Could you check a few things on this model? Use its own coordinates, in mm. A direction names the side the tool comes from. Give positions to 0.01 mm unless a question says otherwise; leave off trailing zeros. Order: outer loops, then holes, each group sorted by start corner. A loop starts at its lowest first (then second) coordinate and runs counter-clockwise, first axis right, second up. Notation, with made-up numbers: M 20,8.25 L 38,8.25 A31 ccw 38,46.25 Z; hole C 2.25,59 d10. An arc over 180 degrees is marked long. Use a Markdown table: item, result. Add a question column.
Item 1: If I drill on L1, parallel to X at y = 0, z = 56.5; L2, parallel to Y at x = -0.25, z = 55.5; L3, parallel to Y at x = 3.1, z = 60, over which ranges is the centre line in solid material (lowest first)? Write a range as from..to.
Item 2: If we mould it in two halves opening along Y, with no side actions, what happens to faces 3 (the face through (-3.253, -0.575, 81.114)), 4 (the face through (-0.867, -3.905, 69.02)), 5 (the face through (3, 1, 140))? For each: released by +Y, released by -Y, zero draft, split by the parting line, or undercut.
Item 3: Suppose I cut it at A-A on x = 0. Write out the boundary of the cut face in (y, z).
Item 4: For faces 1 (the face through (3.037, -0.601, 61.908)), 2 (the face through (3.23, 0.45, 81.07)), which set-ups out of +Z, -Z, +X, -X, +Y, -Y let a thin tool reach every point of the face, with its end or its side?
Item 5: Suppose I cut it at C-C on z = 110. Write out the boundary of the cut face in (x, y), plus the area to 3 significant figures.
Item 6: Suppose I cut it at B-B on z = 82.5. Write out the boundary of the cut face in (x, y).
Item 7: Suppose I cut it at D-D on z = 60. Write out the boundary of the cut face in (x, y), plus the area to 3 significant figures.
Item 8: I'm going to push flat-ended pins straight in: pin 1 Ø1 at (x, z) = (3, 83) entering from -Y; pin 2 Ø3 at (y, z) = (3, 63) entering from -X; pin 3 Ø2 at (y, z) = (3, 81) entering from -X. Where does each tip first touch, or does it pass through?
from build123d import *

# Parameters (mm, degrees)
SKETCH1_R                                  = 4
SKETCH1_R_2                                = 2.9
SHAFT_BOSS_EXTRUDE1_DEPTH                  = 140
PCB_MOUNTINGHOPLES_CUT_EXTRUDE1_DEPTH      = 8.232243507
PCB_MOUNTINGHOPLES_CUT_EXTRUDE1_DEPTH_BACK = 16
SKETCH2_R                                  = 1.5
SKETCH3_R                                  = 2
PCB_CONNECTOR_HOLE_CUT_EXTRUDE2_DEPTH      = 10


with BuildPart() as part:
    # Sketch1 → Shaft Boss-Extrude1 (new body)
    with BuildSketch(Plane.XY):
        Circle(SKETCH1_R)
        Circle(SKETCH1_R_2, mode=Mode.SUBTRACT)
    extrude(amount=SHAFT_BOSS_EXTRUDE1_DEPTH)

    # Sketch2 → PCB Mountinghoples Cut-Extrude1 (cut, two sides: drawn at the far end of the back side and taken through both)
    with BuildSketch(Plane(origin=(0, 0, 0), x_dir=(0, 0, -1), z_dir=(1, 0, 0)).offset(-PCB_MOUNTINGHOPLES_CUT_EXTRUDE1_DEPTH_BACK)):
        with Locations((-82.5, 0)):
            Circle(SKETCH2_R)
        with Locations((-37.5, 0)):
            Circle(SKETCH2_R)
    extrude(amount=PCB_MOUNTINGHOPLES_CUT_EXTRUDE1_DEPTH + PCB_MOUNTINGHOPLES_CUT_EXTRUDE1_DEPTH_BACK, mode=Mode.SUBTRACT)

    # Sketch3 → PCB COnnector Hole Cut-Extrude2 (cut)
    with BuildSketch(Plane(origin=(0, 0, 0), x_dir=(0, 0, -1), z_dir=(1, 0, 0))):
        with Locations(Location((-60, 0, 0), (0, 0, 180))):
            Circle(SKETCH3_R)
    extrude(amount=PCB_CONNECTOR_HOLE_CUT_EXTRUDE2_DEPTH, mode=Mode.SUBTRACT)


solid = part.part
Findings below:
| question | item | result |
|---|---|---|
| 1 | L1 | x = -4..-2.9, 2.9..4 |
| 1 | L2 | y = -3.99..-2.89, 2.89..3.99 |
| 1 | L3 | y = -2.53..-2, 2..2.53 |
| 2 | face 3 | undercut |
| 2 | face 4 | split by the parting line |
| 2 | face 5 | zero draft |
| 3 | outline | M -4,0 L -2.9,0 L -2.9,140 L -4,140 Z; M 2.9,0 L 4,0 L 4,140 L 2.9,140 Z |
| 4 | face 1 | +X |
| 4 | face 2 | +X, -X |
| 5 | outline | C 0,0 d8; hole C 0,0 d5.8 |
| 5 | area | 23.8 mm^2 |
| 6 | outline | M -3.71,-1.5 A4 ccw 3.71,-1.5 L 2.48,-1.5 A2.9 cw -2.48,-1.5 Z; M -3.71,1.5 L -2.48,1.5 A2.9 cw 2.48,1.5 L 3.71,1.5 A4 ccw Z |
| 7 | outline | M 2.1,-2 A2.9 cw long 2.1,2 L 3.46,2 A4 ccw long 3.46,-2 Z |
| 7 | area | 19.1 mm^2 |
| 8 | pin 1 | stops at y = -3.12 |
| 8 | pin 2 | stops at x = -3.71 |
| 8 | pin 3 | stops at x = -3.46 |
